Part model, mm, in its own coordinate system. Face numbers are marked on the shaded views. A direction names the side the tool comes from. Round coordinates to 2 decimals unless told otherwise and drop trailing zeros. Order: outer loops, then holes, each group sorted by start corner. A loop starts at its lowest first (then second) coordinate and runs counter-clockwise, first axis right, second up. Notation, with made-up numbers: (4.25, -38) - (61.25, -38) arc R26 ccw to (61.25, -16) - close; hole circle Ø11 at (25.25, 10.25). An arc over 180 degrees is marked (long way). Answer as a JSON object with one key per item and string values.
```python
from build123d import *

# Parameters (mm, degrees)
BOSS_EXTRUDE1_DEPTH = 11
SKETCH3_R           = 3.5
CUT_EXTRUDE1_DEPTH  = 13
BOSS_EXTRUDE2_DEPTH = 11
SKETCH6_R           = 1.7
CUT_EXTRUDE2_DEPTH  = 50.8
FILLET1_R           = 2.54
FILLET2_R           = 1.27
FILLET3_R           = 1.27
FILLET4_R           = 1.27
FILLET5_R           = 1.27
FILLET6_R           = 1.27
FILLET7_R           = 1.27
SKETCH7_R           = 1.651
SKETCH7_R_2         = 1.7
CUT_EXTRUDE3_DEPTH  = 60.96
FILLET8_R           = 1.27


with BuildPart() as part:
    # Sketch2 → Boss-Extrude1 (new body)
    with BuildSketch(Plane(origin=(0, 0, 0), x_dir=(1, 0, 0), z_dir=(0, 1, 0))):
        Polygon((0, 43), (0, 0), (-20, 0), (-35, -3.5), (-45, -3.5), (-45, 46.5), (-35, 46.5), (-20, 43), align=None)
    extrude(amount=BOSS_EXTRUDE1_DEPTH)

    # Sketch3 → Cut-Extrude1 (cut)
    with BuildSketch(Plane.XZ):
        with Locations(Location((-6.632378844, -5.680552133, 0), (0, 0, 270))):
            Circle(SKETCH3_R)
        with Locations(Location((-6.631542689, -37.680552122, 0), (0, 0, 270))):
            Circle(SKETCH3_R)
    extrude(amount=-CUT_EXTRUDE1_DEPTH, mode=Mode.SUBTRACT)

    # Sketch5 → Boss-Extrude2 (add)
    with BuildSketch(Plane.ZY.offset(45)):
        Polygon((3.5, 11), (3.5, -65.2), (-17.545, -65.2), (-17.545, -2.725115984), (-25.545, -2.725115984), (-25.545, -65.2), (-46.5, -65.2), (-46.5, 11), align=None)
    extrude(amount=BOSS_EXTRUDE2_DEPTH)

    # Sketch6 → Cut-Extrude2 (cut)
    with BuildSketch(Plane(origin=(0, 0, -46.5), x_dir=(-1, 0, 0), z_dir=(0, 0, -1))):
        with Locations(Location((50.5, -6.479893852, 0), (0, 0, 270))):
            Circle(SKETCH6_R)
        with Locations(Location((50.5, -23.36828279, 0), (0, 0, 270))):
            Circle(SKETCH6_R)
        with Locations(Location((50.5, -14.35419589, 0), (0, 0, 270))):
            Circle(SKETCH6_R)
    extrude(amount=-CUT_EXTRUDE2_DEPTH, mode=Mode.SUBTRACT)

    # Fillet1
    fillet1_edges = [part.edges().sort_by_distance(p)[0] for p in [
        (-56, 11, -21.5),
    ]]
    fillet(fillet1_edges, radius=FILLET1_R)

    # Fillet2
    fillet2_edges = [part.edges().sort_by_distance(p)[0] for p in [
        (-45, 0, -21.5),
    ]]
    fillet(fillet2_edges, radius=FILLET2_R)

    # Fillet3
    fillet3_edges = [part.edges().sort_by_distance(p)[0] for p in [
        (0, 5.5, 0),
    ]]
    fillet(fillet3_edges, radius=FILLET3_R)

    # Fillet4
    fillet4_edges = [part.edges().sort_by_distance(p)[0] for p in [
        (0, 5.5, -43),
    ]]
    fillet(fillet4_edges, radius=FILLET4_R)

    # Fillet5
    fillet5_edges = [part.edges().sort_by_distance(p)[0] for p in [
        (-50.5, -65.2, -25.545),
        (-50.5, -65.2, -17.545),
    ]]
    fillet(fillet5_edges, radius=FILLET5_R)

    # Fillet6
    fillet6_edges = [part.edges().sort_by_distance(p)[0] for p in [
        (-56, -65.2, -6.3875),
        (-56, -33.327557992, -25.545),
        (-56, -64.828025612, -25.916974388),
        (-56, -64.828025612, -17.173025612),
        (-56, -65.2, -36.6575),
        (-56, -33.327557992, -17.545),
    ]]
    fillet(fillet6_edges, radius=FILLET6_R)

    # Fillet7
    fillet7_edges = [part.edges().sort_by_distance(p)[0] for p in [
        (-56, -27.735, 3.5),
        (-49.865, -65.2, 3.5),
        (-55.628025612, -64.828025612, 3.5),
        (-49.865, -65.2, -46.5),
        (-55.628025612, -64.828025612, -46.5),
        (-44.23, 11, 3.5),
        (-56, -27.735, -46.5),
        (-44.23, 11, -46.5),
        (-55.256051224, 10.256051224, -46.5),
        (-55.256051224, 10.256051224, 3.5),
    ]]
    fillet(fillet7_edges, radius=FILLET7_R)

    # Sketch7 → Cut-Extrude3 (cut)
    with BuildSketch(Plane(origin=(0, 0, -46.5), x_dir=(-1, 0, 0), z_dir=(0, 0, -1))):
        with Locations((50.5, -60.041602357)):
            Circle(SKETCH7_R)
        with Locations((50.5, -46.740028499)):
            Circle(SKETCH7_R_2)
    extrude(amount=-CUT_EXTRUDE3_DEPTH, mode=Mode.SUBTRACT)

    # Fillet8
    fillet8_edges = [part.edges().sort_by_distance(p)[0] for p in [
        (-45, -65.2, -7.0225),
        (-45, -33.327557992, -25.545),
        (-45, -64.828025612, -25.916974388),
        (-45, -64.828025612, -17.173025612),
        (-45, -65.2, -36.0225),
        (-45, -32.6, 3.5),
        (-45, -64.828025612, 3.128025612),
        (-45, -64.828025612, -46.128025612),
        (-45, -33.327557992, -17.545),
        (-39.365, 0, 3.5),
        (-39.365, 0, -46.5),
        (-45, -32.6, -46.5),
        (-44.628025612, -0.371974388, -46.5),
        (-44.628025612, -0.371974388, 3.5),
    ]]
    fillet(fillet8_edges, radius=FILLET8_R)


solid = part.part
```
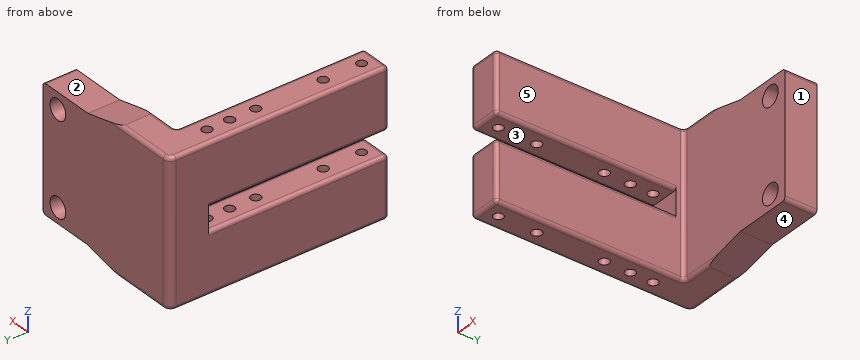
Item 1: Drop flat-ended pins along their axis: P1, Ø3, axis at x = -50.5, y = -6.48, coming from the +Z side; P2, Ø10, axis at x = -10.5, z = -35.5, coming from the -Y side; P3, Ø5.5, axis at x = -6, y = 8, coming from the +Z side; P4, Ø3, axis at x = -53, z = -23.5, coming from the -Y side. Give the stop position or say it passes through.
Taken from the geometry:
{"P1": "through", "P2": "y = 0", "P3": "z = 0", "P4": "y = -2.73"}
Item 2: Cut at A-A (z = -8). Write the cut outline in (x, y).
Taken from the geometry:
{"outline": "(-56, -63.93) arc R1.27 ccw to (-54.73, -65.2) - (-46.27, -65.2) arc R1.27 ccw to (-45, -63.93) - (-45, -1.27) arc R1.27 cw to (-43.73, 0) - (-9.25, 0) - (-9.25, 11) - (-53.46, 11) arc R2.54 ccw to (-56, 8.46) - close; (-4.01, 0) - (0, 0) - (0, 11) - (-4.01, 11) - close; hole circle Ø3.4 at (-50.5, -46.74); hole circle Ø3.4 at (-50.5, -23.37); hole circle Ø3.4 at (-50.5, -14.35); hole circle Ø3.4 at (-50.5, -6.48); hole circle Ø3.3 at (-50.5, -60.04)"}
Item 3: Cut at C-C (x = -39). Write the cut outline in (y, z), plus the area to 3 significant figures.
Taken from the geometry:
{"outline": "(0, -45.23) arc R1.27 ccw to (1.27, -46.5) - (9.73, -46.5) arc R1.27 ccw to (11, -45.23) - (11, 2.23) arc R1.27 ccw to (9.73, 3.5) - (1.27, 3.5) arc R1.27 ccw to (0, 2.23) - close", "area": "549 mm2"}
Item 4: Tool access for the marked faces 1, 2, 3, 4 and 5: list every direction of +Z, -Z, +X, -X, +Y, -Y with a clear straight run to the whole face (end or side of a thin tool).
Taken from the geometry:
{"face 1": "+Z, -Z, +X, +Y, -Y", "face 2": "+Z, +X, +Y, -Y", "face 3": "+X, -X, -Y", "face 4": "-Z, +X, +Y, -Y", "face 5": "+Z, -Z, +X, -Y"}
Item 5: Cut at B-B (y = -57). Write the cut outline in (x, z) (3 decimals), plus the area to 3 significant figures.
Taken from the geometry:
{"outline": "(-56, -45.23) arc R1.27 ccw to (-54.73, -46.5) - (-46.27, -46.5) arc R1.27 ccw to (-45, -45.23) - (-45, -26.815) arc R1.27 ccw to (-46.27, -25.545) - (-54.73, -25.545) arc R1.27 ccw to (-56, -26.815) - close; (-56, -16.275) arc R1.27 ccw to (-54.73, -17.545) - (-46.27, -17.545) arc R1.27 ccw to (-45, -16.275) - (-45, 2.23) arc R1.27 ccw to (-46.27, 3.5) - (-54.73, 3.5) arc R1.27 ccw to (-56, 2.23) - close", "area": "459 mm2"}
Item 6: Cut at D-D (y = -15). Write the cut outline in (x, z) (3 decimals), plus the area to 3 significant figures.
Taken from the geometry:
{"outline": "(-56, -45.23) arc R1.27 ccw to (-54.73, -46.5) - (-52.073, -46.5) - (-52.073, -25.545) - (-54.73, -25.545) arc R1.27 ccw to (-56, -26.815) - close; (-56, -16.275) arc R1.27 ccw to (-54.73, -17.545) - (-52.073, -17.545) - (-52.073, 3.5) - (-54.73, 3.5) arc R1.27 ccw to (-56, 2.23) - close; (-48.927, -46.5) - (-46.27, -46.5) arc R1.27 ccw to (-45, -45.23) - (-45, -26.815) arc R1.27 ccw to (-46.27, -25.545) - (-48.927, -25.545) - close; (-48.927, -17.545) - (-46.27, -17.545) arc R1.27 ccw to (-45, -16.275) - (-45, 2.23) arc R1.27 ccw to (-46.27, 3.5) - (-48.927, 3.5) - close", "area": "327 mm2"}
Item 7: Probe L1, parallel to Y at x = -50.5, z = -33.25; L2, parallel to Z at x = -50.5, y = -38 (3 decimals); L3, parallel to Y at x = -50, z = -30. List the from-to ranges inside material, lowest first. Write a range as from..to.
Taken from the geometry:
{"L1": "-65.2..-61.69, -58.39..-48.44, -45.04..-25.07, -21.67..-16.05, -12.65..-8.18, -4.78..11", "L2": "-46.5..-25.545, -17.545..3.5", "L3": "-65.2..-61.62, -58.47..-48.36, -45.12..-24.99, -21.74..-15.98, -12.73..-8.1, -4.86..11"}
